Autodesk Inventor part; units mm, degrees
ref_plane "Arbeitsebene1" through (0, 0, 180) normal (0, 0, 1) x (1, 0, 0)
ref_plane "YZ Plane" through (0, 0, 0) normal (1, 0, 0) x (0, 1, 0)
ref_plane "XZ Plane" through (0, 0, 0) normal (0, 1, 0) x (-1, 0, 0)
sketch "Skizze1" plane through (0, 0, 0) normal (0, 0, 1) x (1, 0, 0)
  line L0 (-276.5, 0) -> (276.5, 0)
  line L1 (0, -192.5) -> (0, 192.5)
  line L2 (-197.5, 137.5) -> (197.5, 137.5)
  line L3 (197.5, 137.5) -> (197.5, -137.5)
  line L4 (197.5, -137.5) -> (-197.5, -137.5)
  line L5 (-197.5, -137.5) -> (-197.5, 137.5)
  point P0 (0, 0)
  dimension "d0" = 395
  dimension "d1" = 275
extrude "Extrusion1" add sketch "Skizze1" along normal blind 180
sketch "Skizze2" plane through (0, 0, 180) normal (0, 0, 1) x (1, 0, 0)
  line L0 (-195.5, 135.5) -> (195.5, 135.5)
  line L1 (195.5, 135.5) -> (195.5, -135.5)
  line L2 (195.5, -135.5) -> (-195.5, -135.5)
  line L3 (-195.5, -135.5) -> (-195.5, 135.5)
  line L4 (197.5, 137.5) -> (-197.5, 137.5)
  line L5 (197.5, -137.5) -> (197.5, 137.5)
  line L6 (-197.5, -137.5) -> (197.5, -137.5)
  line L7 (-197.5, 137.5) -> (-197.5, -137.5)
  point P0 (0, 0)
  dimension "d4" = 2
  dimension "d5" = 2
  dimension "d6" = 2
  dimension "d7" = 2
extrude "Extrusion2" cut sketch "Skizze2" against normal blind 178 contours L0 L1 L2 L3
ref_plane "Arbeitsebene1" through (0, 0, 180) normal (0, 0, 1) x (1, 0, 0)
sketch "Skizze4" plane through (0, 0, 180) normal (0, 0, 1) x (1, 0, 0)
  line L0 (-207.5, -147.5) -> (207.5, -147.5)
  line L1 (207.5, -147.5) -> (207.5, 147.5)
  line L2 (207.5, 147.5) -> (-207.5, 147.5)
  line L3 (-207.5, 147.5) -> (-207.5, -147.5)
  line L4 (-195.5, -135.5) -> (-195.5, 135.5)
  line L5 (-195.5, 135.5) -> (195.5, 135.5)
  line L6 (195.5, 135.5) -> (195.5, -135.5)
  line L7 (195.5, -135.5) -> (-195.5, -135.5)
  point P0 (0, 0)
  dimension "d17" = 12
  dimension "d18" = 12
  dimension "d19" = 12
  dimension "d20" = 12
extrude "Extrusion4" add sketch "Skizze4" along normal blind 2
sketch "Skizze5" plane through (0, 0, 0) normal (0, 0, -1) x (-1, 0, 0)
  line L0 (-197.5, -137.5) -> (-197.5, 137.5)
  line L1 (-197.5, 137.5) -> (197.5, 137.5)
  circle A0 centre (-147.5, 87.5) radius 15
  point P0 (0, 0)
  dimension "d23" = 50
  dimension "d24" = 50
  dimension "d25" = 30
extrude "Extrusion5" cut sketch "Skizze5" against normal blind 10
sketch "Skizze6" plane through (-195.5, -135.5, 2) normal (0, 1, 0) x (1, 0, 0)
  line L0 (35.8194, -90) -> (175.8194, -90)
  line L1 (175.8194, -90) -> (175.8194, -160)
  line L2 (175.8194, -160) -> (35.8194, -160)
  line L3 (35.8194, -160) -> (35.8194, -90)
  line L4 (391, -180) -> (0, -180)
  point P0 (195.5, 2)
  dimension "d28" = 70
  dimension "d29" = 140
  dimension "d30" = 20
extrude "Extrusion6" cut sketch "Skizze6" against normal blind 10
sketch "Skizze7" plane through (0, 0, 2) normal (0, 0, 1) x (1, 0, 0)
  line L0 (-195.5, -135.5) -> (-195.5, 135.5)
  line L1 (-195.5, 135.5) -> (195.5, 135.5)
  circle A0 centre (-165.5, 105.5) radius 7.5
  point P0 (0, 0)
  dimension "d33" = 30
  dimension "d34" = 30
  dimension "d35" = 15
extrude "Extrusion7" cut sketch "Skizze7" against normal blind 10
sketch "Skizze8" plane through (-195.5, -135.5, 2) normal (0, 1, 0) x (1, 0, 0)
  line L0 (391, 0) -> (0, 0)
  line L1 (391, 0) -> (391, -180)
  circle A0 centre (361, -40) radius 5
  circle A1 centre (331, -40) radius 5
  point P0 (195.5, 2)
  dimension "d38" = 40
  dimension "d39" = 40
  dimension "d40" = 30
  dimension "d41" = 30
  dimension "d42" = 10
  dimension "d43" = 10
extrude "Extrusion8" cut sketch "Skizze8" against normal blind 10
properties part number "Schaltkasten"
For this review, take the finished solid that the model builds, in its own axes (mm). A direction names the side the tool comes from. Round coordinates to 2 decimals unless told otherwise and drop trailing zeros. Loops run counter-clockwise (first coordinate to the right, second up) from the corner with the lowest first, then second, coordinate; pieces in that order, holes last.
(1) Clearance check with flat-ended pins moving along their axes: P1, Ø1, axis at y = -136, z = 143.5, coming from the -X side; P2, Ø1, axis at x = -67.5, y = 84.5, coming from the +Z side; P3, Ø4, axis at x = -41.5, z = 84.5, coming from the -Y side. State where each tip first meets the part, or that it passes through.
Returned:
P1: stops at x = -197.5
P2: stops at z = 2
P3: stops at y = -137.5
(2) We need section D-D (x = 53). Give the boundary of the cut face in (y, z).
Returned:
outline: (-147.5, 180) - (-137.5, 180) - (-137.5, 0) - (137.5, 0) - (137.5, 180) - (147.5, 180) - (147.5, 182) - (135.5, 182) - (135.5, 2) - (-135.5, 2) - (-135.5, 182) - (-147.5, 182) - close
(3) We need section C-C (z = 166.5). Give the boundary of the cut face in (x, y).
Returned:
outline: (-197.5, -137.5) - (197.5, -137.5) - (197.5, 137.5) - (-197.5, 137.5) - close; hole (-195.5, -135.5) - (195.5, -135.5) - (195.5, 135.5) - (-195.5, 135.5) - close
(4) Tool access review of faces 5 (the flat face through (197.5, 2, 89)), 6 (the flat face through (-3, 135.5, 91)), 7 (the flat face through (-16, -141, 180)), 8 (the cylindrical face through (138.188, -136.486, 37.784)), 9 (the flat face through (-197.5, -2, 89)): name each direction out of +Z, -Z, +X, -X, +Y, -Y from which nothing blocks a thin tool from reaching the whole face with its end or side.
Returned:
face 5: -Z, +X, +Y, -Y
face 6: +Z
face 7: -Z
face 8: -Y
face 9: -Z, -X, +Y, -Y
(5) We need section A-A (x = -165.5). Give the boundary of the cut face in (y, z), plus the area to 3 significant figures.
Returned:
outline: (-147.5, 180) - (-137.5, 180) - (-137.5, 0) - (98, 0) - (98, 2) - (-135.5, 2) - (-135.5, 182) - (-147.5, 182) - close; (113, 0) - (137.5, 0) - (137.5, 180) - (147.5, 180) - (147.5, 182) - (135.5, 182) - (135.5, 2) - (113, 2) - close
area: 1,280 mm2
(6) We need section B-B (y = 87.5). Give the boundary of the cut face in (x, z), plus the area to 3 significant figures.
Returned:
outline: (-207.5, 180) - (-197.5, 180) - (-197.5, 0) - (132.5, 0) - (132.5, 2) - (-195.5, 2) - (-195.5, 182) - (-207.5, 182) - close; (162.5, 0) - (197.5, 0) - (197.5, 180) - (207.5, 180) - (207.5, 182) - (195.5, 182) - (195.5, 2) - (162.5, 2) - close
area: 1,490 mm2
(7) Wall thickness on line 1 along X through (y, z) = (-136.65, 42); line 2 along Z through (x, y) = (165.5, -136.2); line 3 along X through (y, z) = (-125.5, 124.5): over which ranges is each line inside the solid? List them lowest first.
Returned:
line 1: x = -197.5 to 130.5, 140.5 to 160.5, 170.5 to 197.5
line 2: z = 0 to 37, 47 to 182
line 3: x = -197.5 to -195.5, 195.5 to 197.5
(8) Mouldability with a two-part tool opening along Y and no side actions: class faces 1 (the flat face through (-3, 137.5, 89)), 2 (the flat face through (195.5, 2, 91)), 3 (the flat face through (-3, 2, 0)), 4 (the flat face through (3, -135.5, 91)) as released by +Y, released by -Y, zero draft, split by the parting line, or undercut.
Returned:
face 1: released by +Y
face 2: undercut
face 3: zero draft
face 4: undercut
